Part model, mm, in its own coordinate system. A direction names the side the tool comes from. Give positions to 0.01 mm unless a question says otherwise; leave off trailing zeros. Write each loop counter-clockwise with the first axis right and the second up, starting at its lowest first coordinate (ties: lowest second). Pieces come first, ordered by that corner, then holes. Notation, with made-up numbers: M 54,79 L 109,79 A10 cw 109,87 Z; hole C 7.25,80 d3. An arc over 180 degrees is marked long. Use CSV: the item, a comma, the result in double quotes. Start each with the question number.
Item 1: Mould opens along X. For faces 3 (the flat face through (-17.5, -15, 0)), 4 (the flat face through (0, 1, 17.5)), 5 (the cylindrical face through (16.07, 1, 0.25)), 6 (the flat face through (0, 0, 8)) say: released by +X, released by -X, zero draft, split by the parting line, or undercut.
Item 2: Pin check, flat tip, straight feed: pin 1 (1.5 mm diameter, centred on x = 4, z = 5.5, fed in from -Y). Stop position of the tip, or through.
Item 3: Cut at D-D (z = -8.5). List the corners of the cut face in (x, y), then the cut area to 3 significant figures.
Item 4: Which spindle directions (+Z, -Z, +X, -X, +Y, -Y) get a long thin tool onto all of the face, cutting with end or side? Do faces 1 (the flat face through (0, 1, -17.5)), 2 (the flat face through (15, -15, 0)). Say none if no direction does.
Item 5: Cut at A-A (y = -4.75). List the corners of the cut face in (x, z).
Item 6: Drill centre lines: line 1 (X direction, y = -6.75, z = 11.5); line 2 (Z direction, x = 0, y = 1.25). Where is each one in solid material? Low to high. Write a range as [from, to].
Autodesk Inventor part; units mm, degrees
ref_plane "YZ Plane" through (0, 0, 0) normal (1, 0, 0) x (0, 1, 0)
ref_plane "XZ Plane" through (0, 0, 0) normal (0, 1, 0) x (-1, 0, 0)
ref_plane "XY Plane" through (0, 0, 0) normal (0, 0, 1) x (1, 0, 0)
sketch "Náčrt2" plane through (0, 0, 0) normal (0, 1, 0) x (-1, 0, 0)
  line L0 (17.5, 17.5) -> (-17.5, 17.5)
  line L1 (-17.5, 17.5) -> (-17.5, -17.5)
  line L2 (-17.5, -17.5) -> (17.5, -17.5)
  line L3 (17.5, -17.5) -> (17.5, 17.5)
  circle A0 centre (0, 0) radius 6.55
  point P0 (17.5, 0)
  point P1 (0, 17.5)
  dimension "d0" = 35
  dimension "d1" = 35
  dimension "d22" = 13.1
extrude "Vysunutí1" add sketch "Náčrt2" along normal blind 2.5
sketch "Náčrt5" plane through (-15, 2.5, -17.5) normal (-1, 0, 0) x (0, -1, 0)
  line L0 (0, 35) -> (0, 0)
  line L1 (0, 0) -> (30, 0)
  line L2 (30, 0) -> (30, 35)
  line L3 (30, 35) -> (0, 35)
edge flange "Obruba2" height 30 angle 90 thickness 2.5 bend radius 2.5 thickness toward (-1, 0, 0) relief tear relief width 2.5 relief depth 1.25 corner gap 2.5 corner form 0 edges at (-17.5, 0, 0) (17.5, 0, 0) wall of the first edge with corners at (-15, 2.5, 17.5) (-15, 2.5, -17.5) (-15, -27.5, -17.5) (-15, -27.5, 17.5)
bend "Ohyb2"
corner "Roh2"
fillet "Zaoblení6" radius 1.25 1 edges at (6.55, 2.5, 0)
fillet "Zaoblení7" radius 1.25 1 edges at (6.55, 0, 0)
equation "\"d29\" = ŠířkaVýštipu"
equation "\"d30\" = HloubkaVýštipu"
equation "\"d31\" = MinimálníZbytek"
equation "\"d32\" = PoloměrOhybu"
equation "\"d35\" = PoloměrOhybu"
equation "\"d36\" = VelikostRohovéhoVýštipu"
equation "\"d37\" = VelikostMezery"
equation "\"d38\" = VelikostJacobihoPoloměru"
equation "\"PoloměrOhybu\" = Tloušťka"
equation "\"ŠířkaVýštipu\" = Tloušťka"
equation "\"HloubkaVýštipu\" = 0.5 * Tloušťka"
equation "\"MinimálníZbytek\" = 2 * Tloušťka"
equation "\"PřechodovýPoloměr\" = PoloměrOhybu"
equation "\"VelikostJacobihoPoloměru\" = PoloměrOhybu"
equation "\"VelikostMezery\" = Tloušťka"
properties part number "DD_KVD_002_11" material "Nerezová ocel"
Worked answers:
1,face 3,"released by -X"
1,face 4,"zero draft"
1,face 5,"released by +X"
1,face 6,"undercut"
2,pin 1,"stops at y = 0.03"
3,outline,"M -17.5,-27.5 L -15,-27.5 L -15,-2.5 A2.5 cw -12.5,0 L 12.5,0 A2.5 cw 15,-2.5 L 15,-27.5 L 17.5,-27.5 L 17.5,-2.5 A5 ccw 12.5,2.5 L -12.5,2.5 A5 ccw -17.5,-2.5 Z"
3,area,"217 mm^2"
4,face 1,"-Z, +X, -X, +Y, -Y"
4,face 2,"+Z, -Z, -Y"
5,outline,"M -17.5,-17.5 L -15,-17.5 L -15,17.5 L -17.5,17.5 Z; M 15,-17.5 L 17.5,-17.5 L 17.5,17.5 L 15,17.5 Z"
6,line 1,"x = [-17.5, -15], [15, 17.5]"
6,line 2,"z = [-17.5, -6.55], [6.55, 17.5]"
